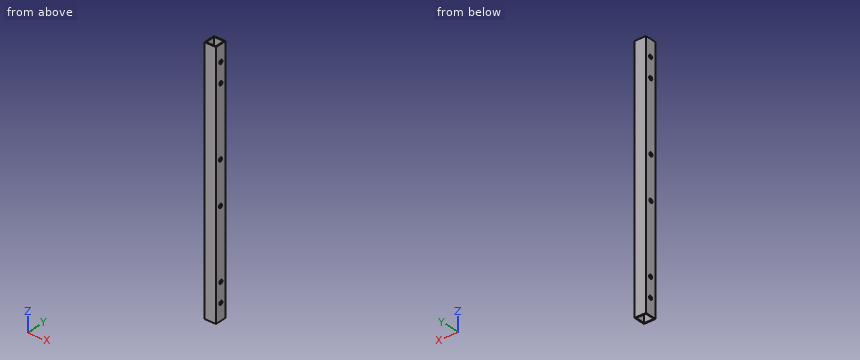
from build123d import *

# Parameters (mm, degrees)
BOSS_EXTRUDE1_START = -34.925
SKETCH1_W           = 38.1
SKETCH1_H           = 38.1
SKETCH1_W_2         = 31.75
SKETCH1_H_2         = 31.75
BOSS_EXTRUDE1_DEPTH = 831.85
SKETCH2_R           = 6.35
CUT_EXTRUDE1_DEPTH  = 799.062634212


with BuildPart() as part:
    # Sketch1 → Boss-Extrude1 (new body)
    with BuildSketch(Plane.XY.offset(BOSS_EXTRUDE1_START)):
        Rectangle(SKETCH1_W, SKETCH1_H)
        Rectangle(SKETCH1_W_2, SKETCH1_H_2, mode=Mode.SUBTRACT)
    extrude(amount=BOSS_EXTRUDE1_DEPTH)

    # Sketch2 → Cut-Extrude1 (cut, through all)
    with BuildSketch(Plane(origin=(19.05, 0, 0), x_dir=(0, 0, -1), z_dir=(1, 0, 0))):
        with Locations((-311.15, -0.905146159)):
            Circle(SKETCH2_R)
        with Locations((-450.85, -0.905146159)):
            Circle(SKETCH2_R)
        with Locations((-679.45, 0.347280154)):
            Circle(SKETCH2_R)
        with Locations((-742.95, 0.347280154)):
            Circle(SKETCH2_R)
        with Locations((-82.55, 0.541693979)):
            Circle(SKETCH2_R)
        with Locations((-19.05, 0.541693979)):
            Circle(SKETCH2_R)
    extrude(amount=-CUT_EXTRUDE1_DEPTH, mode=Mode.SUBTRACT)


solid = part.part
Verification items for the finished model (mm, model axes). Coordinates: 2 decimals unless noted, no trailing zeros. Order: outer loops, then holes, each group sorted by start corner. A loop starts at its lowest first (then second) coordinate and runs counter-clockwise, first axis right, second up. Notation, with made-up numbers: (2, 61.5) -> (52, 61.5) arc R15 ccw to (52, 75.5) -> close; hole circle Ø5 at (-30.75, 75.25). An arc over 180 degrees is marked (long way). Put each result on its own line as item: value. Start each with the question number.
1. Cross-section at B-B, the plane x = -6.5. Record the boundary of the cut face in (y, z) (3 decimals).
2. Cross-section at A-A, the plane z = 33.5. Record the boundary of the cut face in (x, y) (3 decimals), then the cut area to 3 significant figures.
3. Go/stop test with a flat-tipped pin: pin 1 Ø8 at (x, y) = (-8, 11.5) entering from +Z. Record where the tip stops, or that it passes through.
4. Material ranges on L1, parallel to X at y = 5.5, z = 237 (3 decimals); L2, parallel to Y at x = -16.65, z = 82.55, recorded low to high. Write a range as [from, to].
Computed:
1. outline: (-19.05, -34.925) -> (-15.875, -34.925) -> (-15.875, 796.925) -> (-19.05, 796.925) -> close; (15.875, -34.925) -> (19.05, -34.925) -> (19.05, 796.925) -> (15.875, 796.925) -> close
2. outline: (-19.05, -19.05) -> (19.05, -19.05) -> (19.05, 19.05) -> (-19.05, 19.05) -> close; hole (-15.875, -15.875) -> (15.875, -15.875) -> (15.875, 15.875) -> (-15.875, 15.875) -> close
2. area: 444 mm2
3. pin 1: through
4. L1: [-19.05, -15.875], [15.875, 19.05]
4. L2: [-19.05, -5.81], [6.89, 19.05]
